from build123d import *

# Parameters (mm, degrees)
F0_R     = 24.5
F0_R_2   = 15
F0_R_3   = 10
F1_DEPTH = 2
F2_R     = 15
F2_R_2   = 8
F3_DEPTH = 12.3
F4_R     = 10
F4_R_2   = 8
F5_DEPTH = 13.2
F6_D     = 4.4
F6_DEPTH = 14
F6_TIP   = 1.3218933619
F7_R     = 3
F8_DEPTH = 14
F9_SIZE  = 0.5
F10_SIZE = 0.5


with BuildPart() as f1:
    # F0 (on Top) → F1 (new body)
    with BuildSketch(Plane.XY):
        Circle(F0_R)
        Circle(F0_R_2, mode=Mode.SUBTRACT)
        Circle(F0_R_2)
        Circle(F0_R_3, mode=Mode.SUBTRACT)
    extrude(amount=F1_DEPTH)

    # F2 (on face) → F3 (join)
    with BuildSketch(Plane.XY.offset(2)):
        Circle(F2_R)
        Circle(F2_R_2, mode=Mode.SUBTRACT)
    extrude(amount=F3_DEPTH)

    # F4 (on face) → F5 (join)
    with BuildSketch(Plane.XY.offset(2)):
        Circle(F4_R)
        Circle(F4_R_2, mode=Mode.SUBTRACT)
    extrude(amount=-F5_DEPTH)

    # F6
    with Locations(Plane(origin=(0, 0, 0), x_dir=(1, 0, 0), z_dir=(0, 0, -1))):
        with Locations((0, -17.375), (-14.2088220835, 10), (14.2088220835, 10)):
            Hole(F6_D / 2, depth=F6_DEPTH)
            with Locations((0, 0, -(F6_DEPTH + F6_TIP / 2))):  # 118° drill point
                Cone(0, F6_D / 2, F6_TIP, mode=Mode.SUBTRACT)

    # F7 (on face) → F8 (cut)
    with BuildSketch(Plane.XY.offset(14.3)):
        with Locations((0, 7)):
            Circle(F7_R)
        with Locations((-7, 0)):
            Circle(F7_R)
        with Locations((7, 0)):
            Circle(F7_R)
        with Locations((0, -7)):
            Circle(F7_R)
    extrude(amount=-F8_DEPTH, mode=Mode.SUBTRACT)

    # F9
    f9_edges = [f1.edges().sort_by_distance(p)[0] for p in [
        (-10, 0, 14.3),
        (0, 10, 14.3),
        (10, 0, 14.3),
        (0, -10, 14.3),
        (-15, 0, 14.3),
        (-24.5, 0, 2),
        (-10, 0, -11.2),
        (-8, 0, -11.2),
    ]]
    chamfer(f9_edges, length=F9_SIZE)

    # F10
    f10_edges = [f1.edges().sort_by_distance(p)[0] for p in [
        (-24.5, 0, 0),
    ]]
    chamfer(f10_edges, length=F10_SIZE)


solid = f1.part
CAD build for the part. Positions are in the model's coordinates, mm. A direction names the side the tool comes from. Round coordinates to 2 decimals unless told otherwise and drop trailing zeros. Write each loop counter-clockwise with the first axis right and the second up, starting at its lowest first coordinate (ties: lowest second). Pieces come first, ordered by that corner, then holes.
(1) Probe line 1 along Y through (x, z) = (-1, 1.5); line 2 along Y through (x, z) = (0, -4.75); line 3 along Z through (x, y) = (-8, 16.5). List the from-to ranges inside material, lowest first.
(2) Slice it at A-A, the plane z = 4.5. Write the cut outline in (x, y), and give its area (3 significant figures).
(3) Drop flat-ended pins along their axis: P1, Ø0.8, axis at x = -9, y = 0, coming from the +Z side; P2, Ø6, axis at y = 1, z = 0, coming from the -X side; P3, Ø1, axis at x = 4.5, y = 15.5, coming from the -Z side; P4, Ø1, axis at x = -5, z = -7.5, coming from the -Y side. Give the stop position or say it passes through.
(4) Slice it at B-B, the plane x = 0. Count the separate pieces of the cut face and the enclosed holes in it, and give its area (3 significant figures).
(5) Mould opens along Y. For faces 3 (the face through (10.3, 0.3, 0)), 4 (the face through (13.17, 20.66, 0.99)), 5 (the face through (9, 0, 0.3)) say: pulls with the +Y half, pulls with the -Y half, needs draft (parallel to the pull), parting line crosses it, or undercut.
(6) 3-axis set-ups, long thin cutter, end or side, ignore diameter. For faces 1 (the face through (0, -9, 0.3)), 2 (the face through (-15.392, -11.855, 1.014)): which of +Z, -Z, +X, -X, +Y, -Y reach the whole face in a straight line?
(7) Slice it at C-C, the plane z = -8.5. Write the cut outline in (x, y).
From the geometry:
1. line 1: y = -24.48 to -9.83, 9.83 to 15.42, 19.33 to 24.48
1. line 2: y = -10 to -8, 8 to 10
1. line 3: z = 0 to 2
2. outline: circle Ø30 at (0, 0); hole (-7.43, -2.97) arc R8 ccw to (-2.97, -7.43) arc R3 ccw to (2.97, -7.43) arc R8 ccw to (7.43, -2.97) arc R3 ccw to (7.43, 2.97) arc R8 ccw to (2.97, 7.43) arc R3 ccw to (-2.97, 7.43) arc R8 ccw to (-7.43, 2.97) arc R3 ccw to start
2. area: 469 mm2
3. P1: stops at z = 0.3
3. P2: stops at x = -24.5
3. P3: stops at z = 0
3. P4: stops at y = -8.93
4. separate pieces: 3
4. enclosed holes: 0
4. area: 217 mm2
5. face 3: needs draft
5. face 4: parting line crosses it
5. face 5: undercut
6. face 1: +Z
6. face 2: +Z, -Z
7. outline: circle Ø20 at (0, 0); hole circle Ø16 at (0, 0)
